Study the drawing (mm; zero at the part's minimum x, y, z) and answer. Coordinates: 2 decimals unless noted, no trailing zeros. Order: outer loops, then holes, each group sorted by start corner. A loop starts at its lowest first (then second) coordinate and runs counter-clockwise, first axis right, second up. Notation, with made-up numbers: M 77,64 L 105,64 A18 cw 105,84 Z; hole C -12.5,36 d2. An arc over 180 degrees is marked long. Put each result on its own line as item: value.
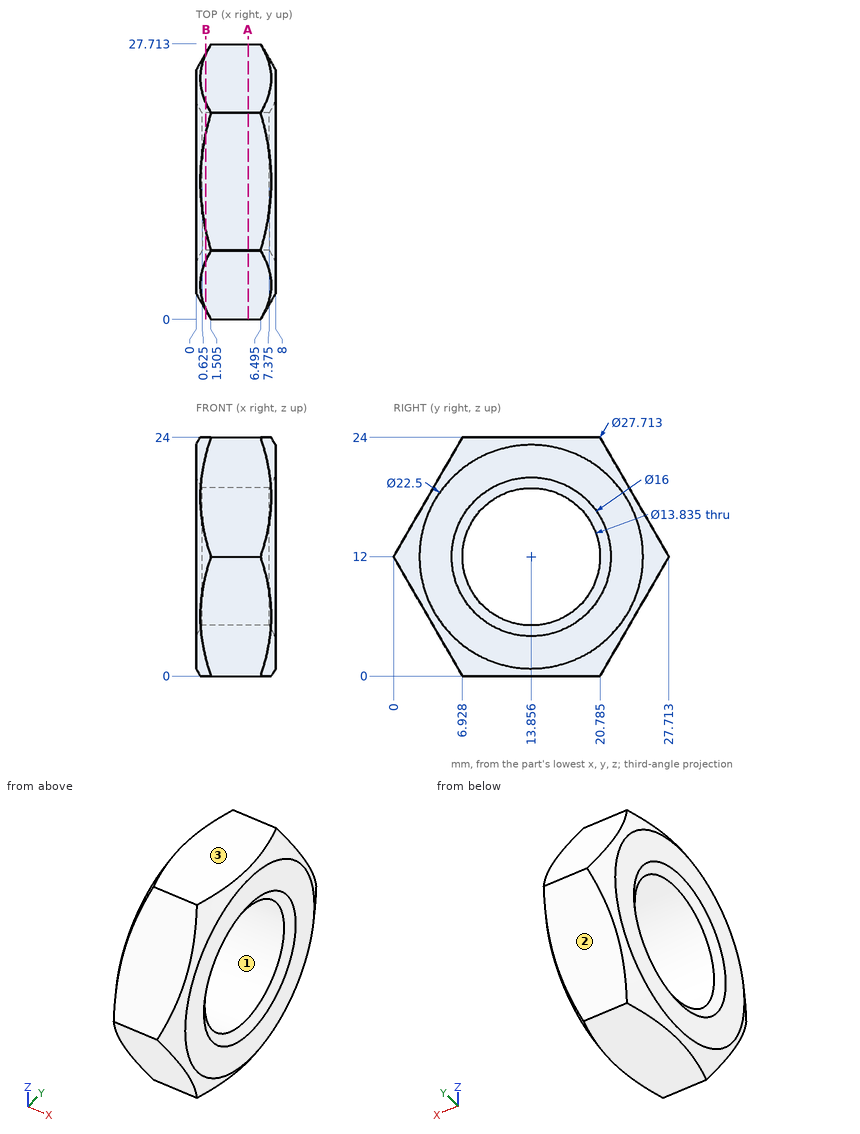
Q1. Consider line 1 along Z through (x, y) = (3.75, 8.75) (1 decimal); line 2 along Z through (x, y) = (7.5, 17) (1 decimal); line 3 along Y through (x, z) = (3.25, 11.25). Determine where each line is inside the solid, lowest interval first.
Answers below:
line 1: z = 0 to 7.3, 16.7 to 24
line 2: z = 0.3 to 5.6, 18.4 to 23.7
line 3: y = 0.43 to 6.98, 20.73 to 27.28
Q2. Given pin 1 (3 mm diameter, centred on x = 3, y = 3.5, fed in from -Z); pin 2 (5 mm diameter, centred on y = 11.5, z = 13, fed in from -X); pin 3 (1 mm diameter, centred on y = 14.5, z = 18.5, fed in from -X); pin 4 (12 mm diameter, centred on y = 5, z = 11.5, fed in from -X), each flat-ended and moving along its own axis, determine where each tip first touches the part or whether it passes through.
Answers below:
pin 1: stops at z = 3.34
pin 2: passes through
pin 3: stops at x = 0.56
pin 4: stops at x = 0
Q3. Find section A-A on x = 5.25. Write down the section's boundary in (y, z) (1 decimal).
Answers below:
outline: M 0,12 L 6.9,0 L 20.8,0 L 27.7,12 L 20.8,24 L 6.9,24 Z; hole C 13.9,12 d13.8
Q4. For a pull along Y with two mould halves and no side action, classify the marked faces 1, 2 and 3 as +Y half, -Y half, draft (parallel to the pull), parting line (faces both ways), or undercut.
Answers below:
face 1: undercut
face 2: +Y half
face 3: draft
Q5. Find section B-B on x = 1. Write down the section's boundary in (y, z) (1 decimal).
Answers below:
outline: M 1,10.3 L 5.9,1.7 A13 ccw 8.9,0 L 18.8,0 A13 ccw 21.8,1.7 L 26.7,10.3 A13 ccw 26.7,13.7 L 21.8,22.3 A13 ccw 18.8,24 L 8.9,24 A13 ccw 5.9,22.3 L 1,13.7 A13 ccw Z; hole C 13.9,12 d13.8
